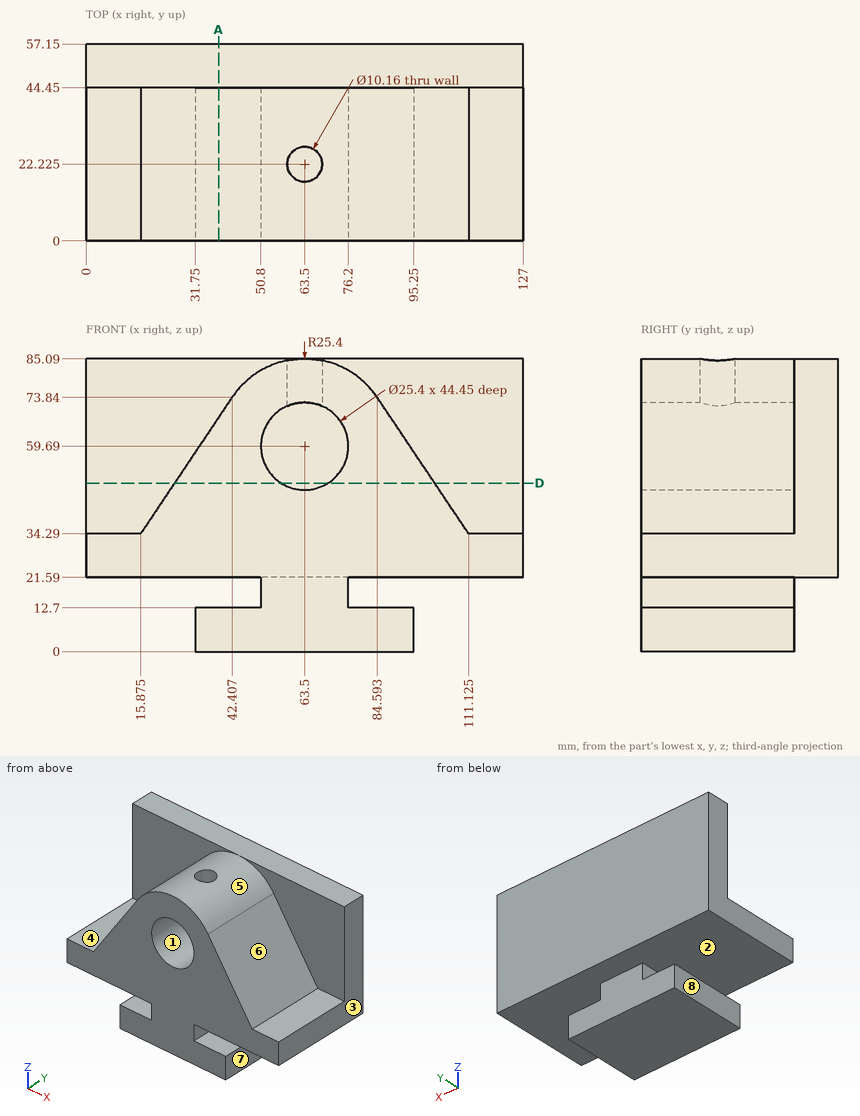
Here's the drawing with two shaded views (mm, measured from the low corner). I have some questions. A direction names the side the tool comes from. Round coordinates to 2 decimals unless told otherwise and drop trailing zeros. Loops run counter-clockwise (first coordinate to the right, second up) from the corner with the lowest first, then second, coordinate; pieces in that order, holes last. Notation, with made-up numbers: (-4, 83) - (46, 83) arc R28 cw to (46, 105) - close; hole circle Ø2 at (66, 53). An arc over 180 degrees is marked (long way). Use CSV: the item, a comma, the result in double quotes.
Item 1: For the marked faces 5, 6, 7 and 8, which set-ups out of +Z, -Z, +X, -X, +Y, -Y let a thin tool reach every point of the face, with its end or its side?
Here are the results:
face 5,"+Z, -Y"
face 6,"+Z, +X, -Y"
face 7,"-Z, +X, +Y, -Y"
face 8,"-Z, -X, +Y, -Y"
Item 2: I need wall thicknesses on L1, parallel to Z at x = 63.5, y = 18; L2, parallel to Y at x = 63, z = 81; L3, parallel to Z at x = 63.5, y = 10.5. Which ranges of each line are inside material? Lowest first, please. Write a range as [from, to].
Here are the results:
L1,"z = [0, 46.99]"
L2,"y = [0, 17.17], [27.28, 57.15]"
L3,"z = [0, 46.99], [72.39, 85.09]"
Item 3: If we mould it in two halves opening along Z, with no side actions, what happens to the marked faces 1, 2, 3 and 4? For each: pulls with the +Z half, pulls with the -Z half, needs draft (parallel to the pull), parting line crosses it, or undercut.
Here are the results:
face 1,"undercut"
face 2,"undercut"
face 3,"needs draft"
face 4,"pulls with the +Z half"
Item 4: Will these pins go through, and if not, where does the flat tip stop? pin 1 (21 mm diameter, centred on x = 39, y = 26, fed in from +Z); pin 2 (12.5 mm diameter, centred on x = 63.5, z = 54.5, fed in from -Y); pin 3 (4 mm diameter, centred on y = 22.5, z = 6.5, fed in from +X).
Here are the results:
pin 1,"stops at z = 80.88"
pin 2,"stops at y = 44.45"
pin 3,"stops at x = 95.25"
Item 5: If we section it at D-D on z = 49: List the corners of the cut face in (x, y) for me.
Here are the results:
outline,"(0, 44.45) - (25.74, 44.45) - (25.74, 0) - (56.64, 0) - (56.64, 44.45) - (70.36, 44.45) - (70.36, 0) - (101.26, 0) - (101.26, 44.45) - (127, 44.45) - (127, 57.15) - (0, 57.15) - close"
Item 6: If we section it at A-A on x = 38.5: List the corners of the cut face in (y, z) for me.
Here are the results:
outline,"(0, 0) - (44.45, 0) - (44.45, 12.7) - (0, 12.7) - close; (0, 21.59) - (57.15, 21.59) - (57.15, 85.09) - (44.45, 85.09) - (44.45, 68.02) - (0, 68.02) - close"
